from build123d import *

# Parameters (mm, degrees)
F0_W     = 107.66001
F0_H     = 107.66
F1_DEPTH = 3.24
F2_W     = 13.195004
F2_H     = 8.148605
F3_DEPTH = 37


with BuildPart() as f1:
    # F0 (on Front) → F1 (new body)
    with BuildSketch(Plane.XZ):
        with Locations((-40.635001, 35.594998)):
            Rectangle(F0_W, F0_H)
    extrude(amount=F1_DEPTH)

    # F2 (on face) → F3 (join)
    with BuildSketch(Plane.XZ.offset(3.24)):
        with Locations((-87.867504, 39.6693)):
            Rectangle(F2_W, F2_H)
        with Locations((6.597502, 39.6693)):
            Rectangle(F2_W, F2_H)
    extrude(amount=F3_DEPTH)


solid = f1.part
Check sheet for the modelled part. Datum: model origin and axes. Units: mm. A direction names the side the tool comes from. Give positions to 0.01 mm unless a question says otherwise; leave off trailing zeros. Write each loop counter-clockwise with the first axis right and the second up, starting at its lowest first coordinate (ties: lowest second). Pieces come first, ordered by that corner, then holes. Notation, with made-up numbers: (-19.5, -17.5) -> (24.5, -17.5) arc R9 cw to (24.5, -5.5) -> close; hole circle Ø7 at (-16.5, 47). An arc over 180 degrees is marked (long way). Write item = value, one per line.
Item 1: Sectioned sample at A-A on y = -13.5. Record the boundary of the cut face in (x, z) (3 decimals), and give its area (3 significant figures).
Output:
outline = (-94.465, 35.595) -> (-81.27, 35.595) -> (-81.27, 43.744) -> (-94.465, 43.744) -> close; (0, 35.595) -> (13.195, 35.595) -> (13.195, 43.744) -> (0, 43.744) -> close
area = 215 mm^2
Item 2: Scan lines: probe 1 along Y at (x, z) = (-14.5, 0); probe 2 along Z at (x, y) = (-81.5, -31.5) (3 decimals). Record each from-to range of solid material in increasing order. Write a range as from..to.
Output:
probe_1 = -3.24..0
probe_2 = 35.595..43.744
Item 3: Sectioned sample at C-C on z = -4. Record the boundary of the cut face in (x, y) (3 decimals).
Output:
outline = (-94.465, -3.24) -> (13.195, -3.24) -> (13.195, 0) -> (-94.465, 0) -> close
Item 4: Tool access check on faces 5 (the flat face through (-41, 0, 36)), 6 (the flat face through (-88, -21, 35.595)), 7 (the flat face through (-88, -21, 43.744)). Record the directions out of +Z, -Z, +X, -X, +Y, -Y that give a thin tool (end or side, any length) a straight path to the whole face; none if there is none.
Output:
face_5 = +Z, -Z, +X, -X, +Y
face_6 = -Z, +X, -X, -Y
face_7 = +Z, +X, -X, -Y
Item 5: Sectioned sample at D-D on x = -65.5. Record the boundary of the cut face in (y, z) (3 decimals), and give its area (3 significant figures).
Output:
outline = (-3.24, -18.235) -> (0, -18.235) -> (0, 89.425) -> (-3.24, 89.425) -> close
area = 349 mm^2
Item 6: Gauge pin test, flat ends, axial feed: pin 1 (10.5 mm diameter, centred on x = 5, y = -25, fed in from +Z); pin 2 (10.5 mm diameter, centred on x = 8, y = -27, fed in from -Z) (3 decimals). Record the tip position at first contact, or that the pin passes through.
Output:
pin_1 = 43.74
pin_2 = 35.595
Item 7: Sectioned sample at B-B on x = -84. Record the boundary of the cut face in (y, z) (3 decimals), and give its area (3 significant figures).
Output:
outline = (-40.24, 35.595) -> (-3.24, 35.595) -> (-3.24, -18.235) -> (0, -18.235) -> (0, 89.425) -> (-3.24, 89.425) -> (-3.24, 43.744) -> (-40.24, 43.744) -> close
area = 650 mm^2
Item 8: Release check for a two-part mould opening along X. For faces 1 (the flat face through (0, -21, 40)), 2 (the flat face through (13.195, -11, 39)), 3 (the flat face through (-81.27, -21, 40)), 4 (the flat face through (-88, -40.24, 40)) record: +X half, -X half, draft (parallel to the pull), parting line (faces both ways), or undercut.
Output:
face_1 = undercut
face_2 = +X half
face_3 = undercut
face_4 = draft
